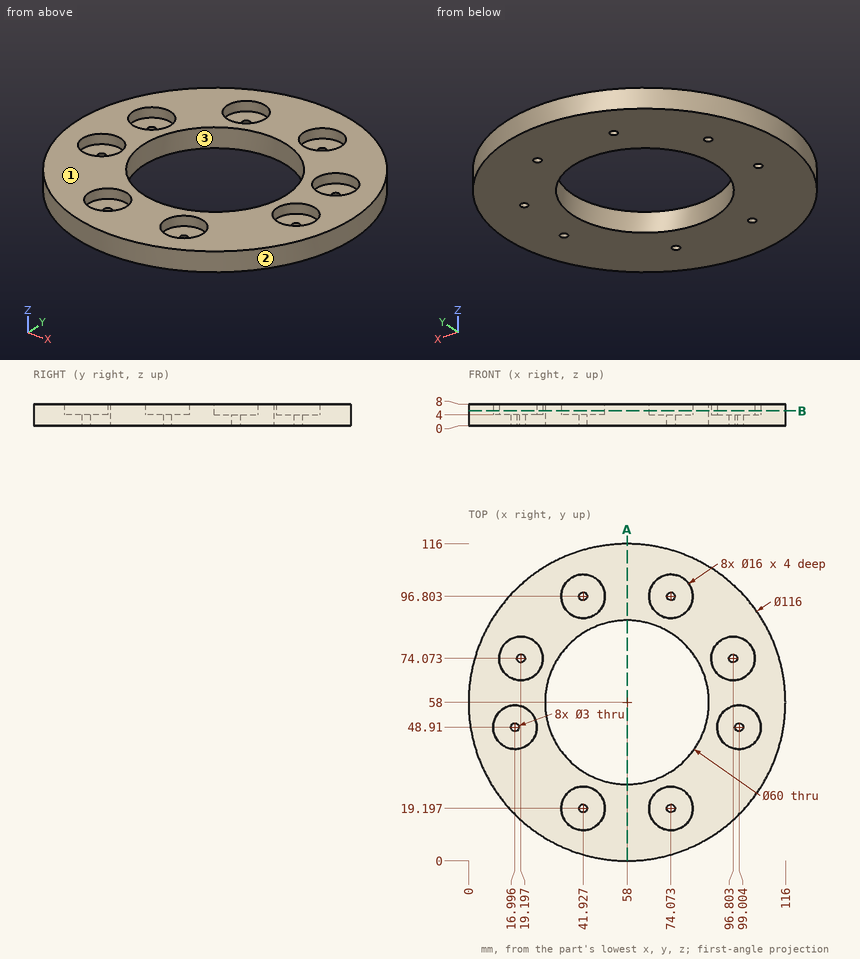
Source: three-view drawing plus pictorial views. Frame: mm from the lowest corner of the part. Give positions to 0.01 mm unless a question says otherwise; leave off trailing zeros. Order: outer loops, then holes, each group sorted by start corner. A loop starts at its lowest first (then second) coordinate and runs counter-clockwise, first axis right, second up. Notation, with made-up numbers: M -3.75,23.5 L 50.25,23.5 A17 ccw 50.25,45.5 Z; hole C 41.5,82 d4. An arc over 180 degrees is marked long. One line per question, with ' | ' between items. Start each with the question number.
1. Pull-direction query (X, two-part tool) for the marked faces 1, 2 and 3; classes: released by +X, released by -X, zero draft, split by the parting line, or undercut.
2. First-contact query: pin 1 Ø5 at (x, y) = (42, 99) entering from +Z; pin 2 Ø17.5 at (x, y) = (15.5, 72) entering from +Z; pin 3 Ø4 at (x, z) = (12.5, 2.5) entering from +Y (1 decimal); pin 4 Ø3 at (y, z) = (104.5, 5) entering from +X. Flat tips, straight axial feed; report the tip coordinate or a pass-through.
3. Material intervals for probe 1 along Y at (x, z) = (58, 2.5); probe 2 along X at (y, z) = (16, 4.5) (1 decimal); probe 3 along X at (y, z) = (94.5, 7) (1 decimal), sorted ascending. Write a range as [from, to].
4. Section query A-A (x = 58). Return the cut outline in (y, z), and give its area (3 significant figures).
5. Section query B-B (z = 5.5). Count the separate pieces of the cut face and the enclosed holes in it, and give its area (3 significant figures).
Here are the results:
1) face 1: zero draft | face 2: split by the parting line | face 3: undercut
2) pin 1: z = 4 | pin 2: z = 8 | pin 3: y = 96.4 | pin 4: x = 94.59
3) probe 1: [0, 28], [88, 116] | probe 2: [18, 34.6], [49.3, 66.7], [81.4, 98] | probe 3: [12.9, 34.3], [49.6, 66.4], [81.7, 103.1]
4) outline: M 0,0 L 28,0 L 28,8 L 0,8 Z; M 88,0 L 116,0 L 116,8 L 88,8 Z | area: 448 mm²
5) separate pieces: 1 | enclosed holes: 9 | area: 6,130 mm²
